from build123d import *

# Parameters (mm, degrees)
FILLET_1_R = 0.6
FILLET_2_R = 0.5


with BuildPart() as part:
    # 草图2 → 旋转1 (revolve)
    with BuildSketch(Plane.XY, mode=Mode.PRIVATE) as revolve_1_sk:
        Polygon((0, 0), (4.5, 0), (4.5, -3.9), (5.5, -3.9), (5.5, -5), (0, -5), align=None)
    revolve(revolve_1_sk.sketch.rotate(Axis((-5, 0, 0), (0, -1, 0)), 180), axis=Axis((-5, 0, 0), (0, -1, 0)))

    # 圆角1
    fillet_1_edges = [part.edges().sort_by_distance(p)[0] for p in [
        (4.5, 0, 0),
    ]]
    fillet(fillet_1_edges, radius=FILLET_1_R)

    # 圆角2
    fillet_2_edges = [part.edges().sort_by_distance(p)[0] for p in [
        (0, 0, 0),
    ]]
    fillet(fillet_2_edges, radius=FILLET_2_R)


solid = part.part
CAD build for the part. Positions are in the model's coordinates, mm. A direction names the side the tool comes from. Round coordinates to 2 decimals unless told otherwise and drop trailing zeros. Order: outer loops, then holes, each group sorted by start corner. A loop starts at its lowest first (then second) coordinate and runs counter-clockwise, first axis right, second up. Notation, with made-up numbers: (-16.75, -4.5) - (13.25, -4.5) arc R20 cw to (13.25, 34.5) - close; hole circle Ø11 at (-16, -4.5). An arc over 180 degrees is marked (long way). Return JSON: item names as keys, results as strings.
(1) Cut at C-C (y = -1.2). Give the cut face in (x, z), then the cut area to 3 significant figures.
Answer key:
{"outline": "circle Ø19 at (-5, 0); hole circle Ø10 at (-5, 0)", "area": "205 mm^2"}
(2) Cut at B-B (z = 0). Give the cut face in (x, y).
Answer key:
{"outline": "(-15.5, -5) - (-10, -5) - (-10, -0.5) arc R0.5 ccw to (-10.5, 0) - (-13.9, 0) arc R0.6 ccw to (-14.5, -0.6) - (-14.5, -3.9) - (-15.5, -3.9) - close; (0, -5) - (5.5, -5) - (5.5, -3.9) - (4.5, -3.9) - (4.5, -0.6) arc R0.6 ccw to (3.9, 0) - (0.5, 0) arc R0.5 ccw to (0, -0.5) - close"}
(3) Pull direction X, two halves, no side cores. Call faces 3 (the face through (-10, -5, 2)), 4 (the face through (2.54, -2.27, 5.78)), 5 (the face through (0, -3, 0)): +X half, -X half, draft (parallel to the pull), parting line (faces both ways), or undercut.
Answer key:
{"face 3": "draft", "face 4": "parting line", "face 5": "undercut"}
(4) Cut at A-A (x = -5). Give the cut face in (y, z), then the cut area to 3 significant figures.
Answer key:
{"outline": "(-5, -10.5) - (-3.9, -10.5) - (-3.9, -9.5) - (-0.6, -9.5) arc R0.6 ccw to (0, -8.9) - (0, -5.5) arc R0.5 ccw to (-0.5, -5) - (-5, -5) - close; (-5, 5) - (-0.5, 5) arc R0.5 ccw to (0, 5.5) - (0, 8.9) arc R0.6 ccw to (-0.6, 9.5) - (-3.9, 9.5) - (-3.9, 10.5) - (-5, 10.5) - close", "area": "46.9 mm^2"}
(5) Tool access for faces 1 (the face through (-3.63, -4.46, -10.41)), 2 (the face through (-10, -3.9, 9)): list every direction of +Z, -Z, +X, -X, +Y, -Y with a clear straight run to the whole face (end or side of a thin tool).
Answer key:
{"face 1": "+Y, -Y", "face 2": "+Y"}
(6) Pin check, flat tips, straight feed: pin 1 Ø1 at (y, z) = (-0.5, -5) entering from -X; pin 2 Ø2 at (y, z) = (-3, -4.5) entering from +X. Stop position of each tip, or through.
Answer key:
{"pin 1": "stops at x = -13.36", "pin 2": "stops at x = 4.68"}
(7) Cut at D-D (y = -4.35). Give the cut face in (x, z).
Answer key:
{"outline": "circle Ø21 at (-5, 0); hole circle Ø10 at (-5, 0)"}
(8) Wall check: probe 1 along Z at (x, y) = (-5, -1.8); probe 2 along Z at (x, y) = (-5, -4.05); probe 3 along X at (y, z) = (-3, 3.75). Give the ranges that are in metal, low to high. Write a range as from..to.
Answer key:
{"probe 1": "z = -9.5..-5, 5..9.5", "probe 2": "z = -10.5..-5, 5..10.5", "probe 3": "x = -13.73..-8.31, -1.69..3.73"}
